Check sheet for the modelled part. Datum: model origin and axes. Units: mm. A direction names the side the tool comes from. Give positions to 0.01 mm unless a question says otherwise; leave off trailing zeros. Loops run counter-clockwise (first coordinate to the right, second up) from the corner with the lowest first, then second, coordinate; pieces in that order, holes last. Notation, with made-up numbers: (-26, 56.25) -> (20, 56.25) arc R21 ccw to (20, 70.25) -> close; hole circle Ø1 at (32.5, -0.75). An arc over 180 degrees is marked (long way). Answer as CSV lines item,"result". Start each with the question number.
(1) Section check B-B on x = 0. Enter the section's corners in (y, z).
(2) Material ranges on line 1 (Z direction, x = 0, y = -1.45); line 2 (Y direction, x = -4.5, z = 4.5); line 3 (Z direction, x = -2, y = 1), recorded low to high. Write a range as from..to.
(3) Release check for a two-part mould opening along X. For faces 5 (the face through (0, 2, 8)), 6 (the face through (5, -2, 9)), 7 (the face through (-5, -2, 9)), 8 (the face through (0.08, -1.37, 15.55)) record: pulls with the +X half, pulls with the -X half, needs draft (parallel to the pull), parting line crosses it, or undercut.
(4) Access from +Z, -Z, +X, -X, +Y, -Y to the whole of each face (thin tool, end or side, straight path). Record for faces 1 (the face through (1, -0.5, 2)), 2 (the face through (0, 3.5, 10)), 3 (the face through (0, 2, 12)), 4 (the face through (0, -3, 12)).
(5) Section check D-D on z = 16.75. Enter the section's corners in (x, y), plus the area to 3 significant figures.
(6) Section check C-C on y = -2.5. Enter the section's corners in (x, z), plus the area to 3 significant figures.
(7) Section check A-A on z = 4. Enter the section's corners in (x, y), plus the area to 3 significant figures.
(8) Gauge pin test, flat ends, axial feed: pin 1 Ø1 at (x, y) = (-2, 1.5) entering from +Z; pin 2 Ø2.5 at (x, z) = (-1.5, 6) entering from +Y; pin 3 Ø1.5 at (x, y) = (3.5, 2) entering from -Z. Record the tip position at first contact, or that the pin passes through.
from build123d import *

# Parameters (mm, degrees)
F0_W     = 10
F0_H     = 7
F1_DEPTH = 19
F2_W     = 10
F2_H     = 4
F3_DEPTH = 7
F4_R     = 2
F5_DEPTH = 7.001
F6_W     = 10
F6_H     = 8
F7_DEPTH = 4


with BuildPart() as f1:
    # F0 (on Top) → F1 (new body)
    with BuildSketch(Plane.XY):
        Rectangle(F0_W, F0_H)
    extrude(amount=F1_DEPTH)

    # F2 (on face) → F3 (cut)
    with BuildSketch(Plane.XY.offset(19)):
        with BuildLine():
            Line((-4.921189, -3.5), (4.921189, -3.5))
            ThreePointArc((4.921189, -3.5), (0, -1.37), (-4.921189, -3.5))
        make_face()
        with Locations((0, 1.5)):
            Rectangle(F2_W, F2_H)
    extrude(amount=-F3_DEPTH, mode=Mode.SUBTRACT)

    # F4 (on face) → F5 (cut, through all)
    with BuildSketch(Plane.XZ.offset(3.5)):
        with Locations((0, 4)):
            Circle(F4_R)
    extrude(amount=-F5_DEPTH, mode=Mode.SUBTRACT)

    # F6 (on face) → F7 (cut)
    with BuildSketch(Plane(origin=(0, 3.5, 0), x_dir=(-1, 0, 0), z_dir=(0, 1, 0))):
        with Locations((0, 4)):
            Rectangle(F6_W, F6_H)
    extrude(amount=-F7_DEPTH, mode=Mode.SUBTRACT)


solid = f1.part
Working result:
1,outline,"(-3.5, 0) -> (-0.5, 0) -> (-0.5, 2) -> (-3.5, 2) -> close; (-3.5, 6) -> (-0.5, 6) -> (-0.5, 8) -> (3.5, 8) -> (3.5, 12) -> (-0.5, 12) -> (-0.5, 19) -> (-1.37, 19) -> (-1.37, 12) -> (-3.5, 12) -> close"
2,line 1,"z = 0..2, 6..12"
2,line 2,"y = -3.5..-0.5"
2,line 3,"z = 8..12"
3,face 5,"needs draft"
3,face 6,"pulls with the +X half"
3,face 7,"pulls with the -X half"
3,face 8,"undercut"
4,face 1,"-Z, +X, -X, +Y"
4,face 2,"+Z, -Z, +X, -X, +Y"
4,face 3,"+Z, +X, -X, +Y"
4,face 4,"+Z, -Y"
5,outline,"(-5, -3.5) -> (-4.92, -3.5) arc R6.75 cw to (4.92, -3.5) -> (5, -3.5) -> (5, -0.5) -> (-5, -0.5) -> close"
5,area,"15.5 mm^2"
6,outline,"(-5, 0) -> (5, 0) -> (5, 19) -> (3.74, 19) -> (3.74, 12) -> (-3.74, 12) -> (-3.74, 19) -> (-5, 19) -> close; hole circle Ø4 at (0, 4)"
6,area,"125 mm^2"
7,outline,"(-5, -3.5) -> (-2, -3.5) -> (-2, -0.5) -> (-5, -0.5) -> close; (2, -3.5) -> (5, -3.5) -> (5, -0.5) -> (2, -0.5) -> close"
7,area,"18.0 mm^2"
8,pin 1,"stops at z = 12"
8,pin 2,"stops at y = -0.5"
8,pin 3,"stops at z = 8"
